Could you check a few things on this model? Use its own coordinates, in mm. A direction names the side the tool comes from. Coordinates: 2 decimals unless noted, no trailing zeros. Loops run counter-clockwise (first coordinate to the right, second up) from the corner with the lowest first, then second, coordinate; pieces in that order, holes last.
from build123d import *

# Parameters (mm, degrees)
SKETCH_1_R          = 15.45
EXTRUDE_1_DEPTH     = 13.5
SKETCH_2_R          = 17.5
EXTRUDE_2_DEPTH     = 2.5
EXTRUDE_START       = 2.5
SKETCH_3_R          = 17.5
EXTRUDE_3_DEPTH     = 2.5
SKETCH_4_R          = 3
CUT_EXTRUDE_1_DEPTH = 41.453677212


with BuildPart() as part:
    # 草图1 → 凸台-拉伸1 (new, symmetric)
    with BuildSketch(Plane(origin=(0, 0, 0), x_dir=(1, 0, 0), z_dir=(0, 1, 0))):
        with Locations(Location((0, 0, 0), (0, 0, 270))):
            Circle(SKETCH_1_R)
    extrude(amount=EXTRUDE_1_DEPTH, both=True)

    # 草图2 → 凸台-拉伸2 (add)
    with BuildSketch(Plane(origin=(0, 13.5, 0), x_dir=(1, 0, 0), z_dir=(0, 1, 0))):
        with Locations(Location((0, 0, 0), (0, 0, 270))):
            Circle(SKETCH_2_R)
    extrude(amount=EXTRUDE_2_DEPTH)

    # 草图3 → 凸台-拉伸3 (add)
    with BuildSketch(Plane.XZ.offset(13.5).offset(EXTRUDE_START)):
        with Locations(Location((0, 0, 0), (0, 0, 90))):
            Circle(SKETCH_3_R)
    extrude(amount=-EXTRUDE_3_DEPTH)

    # 草图4 → 切除-拉伸1 (cut, through all)
    with BuildSketch(Plane(origin=(0, 16, 0), x_dir=(1, 0, 0), z_dir=(0, 1, 0))):
        with Locations(Location((0, 0, 0), (0, 0, 270))):
            Circle(SKETCH_4_R)
    extrude(amount=-CUT_EXTRUDE_1_DEPTH, mode=Mode.SUBTRACT)


solid = part.part
1) Imagine slicing it at A-A on x = 0. List the corners of the cut face in (y, z) for me, plus the area to 3 significant figures.
2) For faces 1 (the cylindrical face through (10.648, -14.768, -13.887)), 2 (the flat face through (-12, 13.5, 10)), which set-ups out of +Z, -Z, +X, -X, +Y, -Y let a thin tool reach every point of the face, with its end or its side?
3) Will these pins go through, and if not, where does the flat tip stop? pin 1 (4 mm diameter, centred on y = 0, z = -10, fed in from -X); pin 2 (10 mm diameter, centred on x = 7, y = 9.5, fed in from +Z); pin 3 (4 mm diameter, centred on y = -8.5, z = -13.5, fed in from +X); pin 4 (3.5 mm diameter, centred on x = 0, z = 0, fed in from +Y).
4) We'd pull the mould along X, two halves only. Please class faces 3 (the cylindrical face through (0.9, 0.22, 2.86)), 4 (the flat face through (-4, 16, 0)), 5 (the cylindrical face through (-9.4, 0.19, -12.26)): released by +X, released by -X, zero draft, split by the parting line, or undercut.
5) Imagine slicing it at B-B on z = 0. List the corners of the cut face in (x, y) for me, plus the area to 3 significant figures.
6) Imagine slicing it at C-C on y = 8. List the corners of the cut face in (x, z) for me, plus the area to 3 significant figures.
7) Imagine slicing it at D-D on z = 6. List the corners of the cut face in (x, y) for me, plus the area to 3 significant figures.
8) If I drill on L1, parallel to X at y = -5, z = 0; L2, parallel to Y at x = 15, z = -7.5; L3, parallel to Z at x = -1, y = 7, over which ranges is the centre line in solid material (lowest first)?
Solved:
1. outline: (-16, -17.5) - (-13.5, -17.5) - (-13.5, -15.45) - (13.5, -15.45) - (13.5, -17.5) - (16, -17.5) - (16, -3) - (-16, -3) - close; (-16, 3) - (16, 3) - (16, 17.5) - (13.5, 17.5) - (13.5, 15.45) - (-13.5, 15.45) - (-13.5, 17.5) - (-16, 17.5) - close
1. area: 817 mm2
2. face 1: +Y, -Y
2. face 2: none
3. pin 1: stops at x = -13.22
3. pin 2: stops at z = 17.04
3. pin 3: stops at x = 10.32
3. pin 4: passes through
4. face 3: undercut
4. face 4: zero draft
4. face 5: split by the parting line
5. outline: (-17.5, -16) - (-3, -16) - (-3, 16) - (-17.5, 16) - (-17.5, 13.5) - (-15.45, 13.5) - (-15.45, -13.5) - (-17.5, -13.5) - close; (3, -16) - (17.5, -16) - (17.5, -13.5) - (15.45, -13.5) - (15.45, 13.5) - (17.5, 13.5) - (17.5, 16) - (3, 16) - close
5. area: 817 mm2
6. outline: circle Ø30.9 at (0, 0); hole circle Ø6 at (0, 0)
6. area: 722 mm2
7. outline: (-16.44, -16) - (16.44, -16) - (16.44, -13.5) - (14.24, -13.5) - (14.24, 13.5) - (16.44, 13.5) - (16.44, 16) - (-16.44, 16) - (-16.44, 13.5) - (-14.24, 13.5) - (-14.24, -13.5) - (-16.44, -13.5) - close
7. area: 933 mm2
8. L1: x = -15.45 to -3, 3 to 15.45
8. L2: y = -16 to -13.5, 13.5 to 16
8. L3: z = -15.42 to -2.83, 2.83 to 15.42
